Check sheet for the modelled part. Datum: model origin and axes. Units: mm. Face numbers are marked on the shaded views. A direction names the side the tool comes from. Coordinates: 2 decimals unless noted, no trailing zeros. Loops run counter-clockwise (first coordinate to the right, second up) from the corner with the lowest first, then second, coordinate; pieces in that order, holes last.
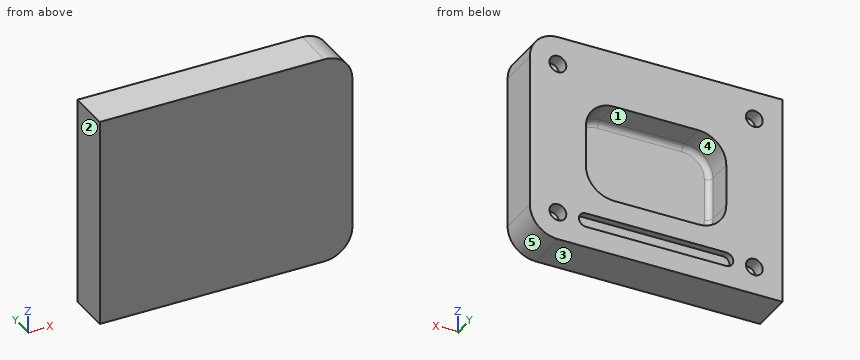
```python
from build123d import *

# Parameters (mm, degrees)
SKETCH1_W                  = 180
SKETCH1_H                  = 150
BOSS_EXTRUDE1_DEPTH        = 30
F_16_0MM_DOWEL_HOLE1_D     = 12
F_16_0MM_DOWEL_HOLE1_DEPTH = 10
F_16_0MM_DOWEL_HOLE1_TIP   = 3.605163714
SKETCH5_W                  = 100
SKETCH5_H                  = 70
CUT_EXTRUDE1_DEPTH         = 22
FILLET1_R                  = 20
FILLET2_R                  = 20
CUT_EXTRUDE2_DEPTH         = 5
FILLET3_R                  = 4


with BuildPart() as part:
    # Sketch1 → Boss-Extrude1 (new body)
    with BuildSketch(Plane(origin=(0, 0, 0), x_dir=(1, 0, 0), z_dir=(0, 1, 0))):
        Rectangle(SKETCH1_W, SKETCH1_H)
    extrude(amount=BOSS_EXTRUDE1_DEPTH)

    # Ø16.0mm Dowel Hole1
    with Locations(Plane(origin=(-70, 30, 55), x_dir=(0, 0, 1), z_dir=(0, 1, 0))):
        with Locations((0, 0), (-110, 0), (-110, 140), (0, 140)):
            Hole(F_16_0MM_DOWEL_HOLE1_D / 2, depth=F_16_0MM_DOWEL_HOLE1_DEPTH)
            with Locations((0, 0, -(F_16_0MM_DOWEL_HOLE1_DEPTH + F_16_0MM_DOWEL_HOLE1_TIP / 2))):  # 118° drill point
                Cone(0, F_16_0MM_DOWEL_HOLE1_D / 2, F_16_0MM_DOWEL_HOLE1_TIP, mode=Mode.SUBTRACT)

    # Sketch5 → Cut-Extrude1 (cut)
    with BuildSketch(Plane(origin=(0, 30, 0), x_dir=(1, 0, 0), z_dir=(0, 1, 0))):
        Rectangle(SKETCH5_W, SKETCH5_H)
    extrude(amount=-CUT_EXTRUDE1_DEPTH, mode=Mode.SUBTRACT)

    # Fillet1
    fillet1_edges = [part.edges().sort_by_distance(p)[0] for p in [
        (50, 19, -35),
        (-50, 19, -35),
        (-50, 19, 35),
        (50, 19, 35),
    ]]
    fillet(fillet1_edges, radius=FILLET1_R)

    # Fillet2
    fillet2_edges = [part.edges().sort_by_distance(p)[0] for p in [
        (90, 15, 75),
        (90, 15, -75),
    ]]
    fillet(fillet2_edges, radius=FILLET2_R)

    # Sketch6 → Cut-Extrude2 (cut)
    with BuildSketch(Plane(origin=(0, 30, 0), x_dir=(1, 0, 0), z_dir=(0, 1, 0))):
        with BuildLine():
            Line((-50, 60), (50, 60))
            ThreePointArc((50, 60), (55, 55), (50, 50))
            Line((50, 50), (-50, 50))
            ThreePointArc((-50, 50), (-55, 55), (-50, 60))
        make_face()
    extrude(amount=-CUT_EXTRUDE2_DEPTH, mode=Mode.SUBTRACT)

    # Fillet3
    fillet3_edges = [part.edges().sort_by_distance(p)[0] for p in [
        (50, 8, 0),
        (0, 8, 35),
        (0, 8, -35),
        (-50, 8, 0),
        (-44.142135624, 8, -29.142135624),
        (44.142135624, 8, -29.142135624),
        (-44.142135624, 8, 29.142135624),
        (44.142135624, 8, 29.142135624),
    ]]
    fillet(fillet3_edges, radius=FILLET3_R)


solid = part.part
```
1) Mould release check, pull along X, two halves, no side actions. Record for the marked faces 1, 2 and 3: +X half, -X half, draft (parallel to the pull), parting line (faces both ways), or undercut.
Answer sheet:
face 1: undercut
face 2: -X half
face 3: draft
2) Section check B-B on x = 23. Enter the section's corners in (y, z), plus the area to 3 significant figures.
Answer sheet:
outline: (0, -75) - (30, -75) - (30, -60) - (25, -60) - (25, -50) - (30, -50) - (30, -35) - (12, -35) arc R4 cw to (8, -31) - (8, 31) arc R4 cw to (12, 35) - (30, 35) - (30, 75) - (0, 75) - close
area: 2,920 mm2
3) Scan lines: line 1 (Z direction, x = 70, y = 26.5); line 2 (X direction, y = 25, z = 55); line 3 (Z direction, x = 4.5, y = 27.75). Record each from-to range of solid material in increasing order.
Answer sheet:
line 1: z = -75 to -61, -49 to 49, 61 to 75
line 2: x = -90 to -76, -64 to 64, 76 to 90
line 3: z = -75 to -60, -50 to -35, 35 to 75
4) Section check A-A on y = 22. Enter the section's corners in (x, z), plus the area to 3 significant figures.
Answer sheet:
outline: (-90, -75) - (70, -75) arc R20 ccw to (90, -55) - (90, 55) arc R20 ccw to (70, 75) - (-90, 75) - close; hole circle Ø12 at (-70, -55); hole circle Ø12 at (-70, 55); hole (-50, -15) arc R20 ccw to (-30, -35) - (30, -35) arc R20 ccw to (50, -15) - (50, 15) arc R20 ccw to (30, 35) - (-30, 35) arc R20 ccw to (-50, 15) - close; hole circle Ø12 at (70, -55); hole circle Ø12 at (70, 55)
area: 19,700 mm2
5) Depth check by flat-ended pin: pin 1 (3 mm diameter, centred on x = -27, z = -54.5, fed in from +Y). Enter the tip coordinate at first touch or a pass-through.
Answer sheet:
pin 1: stops at y = 25
6) Set-up check for the marked faces 4 and 5: record each of +Z, -Z, +X, -X, +Y, -Y from which the full face is reachable in a straight line by a thin tool's end or side.
Answer sheet:
face 4: +Y
face 5: -Z, +X, +Y, -Y
